Input: dimensioned drawing with shaded views. Units: mm. Origin: part minimum x, y, z. Coordinates: 2 decimals unless noted, no trailing zeros. Loops run counter-clockwise (first coordinate to the right, second up) from the corner with the lowest first, then second, coordinate; pieces in that order, holes last. Notation, with made-up numbers: M 27.25,58.5 L 81.25,58.5 A17 ccw 81.25,68.5 Z; hole C 47,17.25 d8. An arc over 180 degrees is marked long. Write item = value, one per line. Start each with the question number.
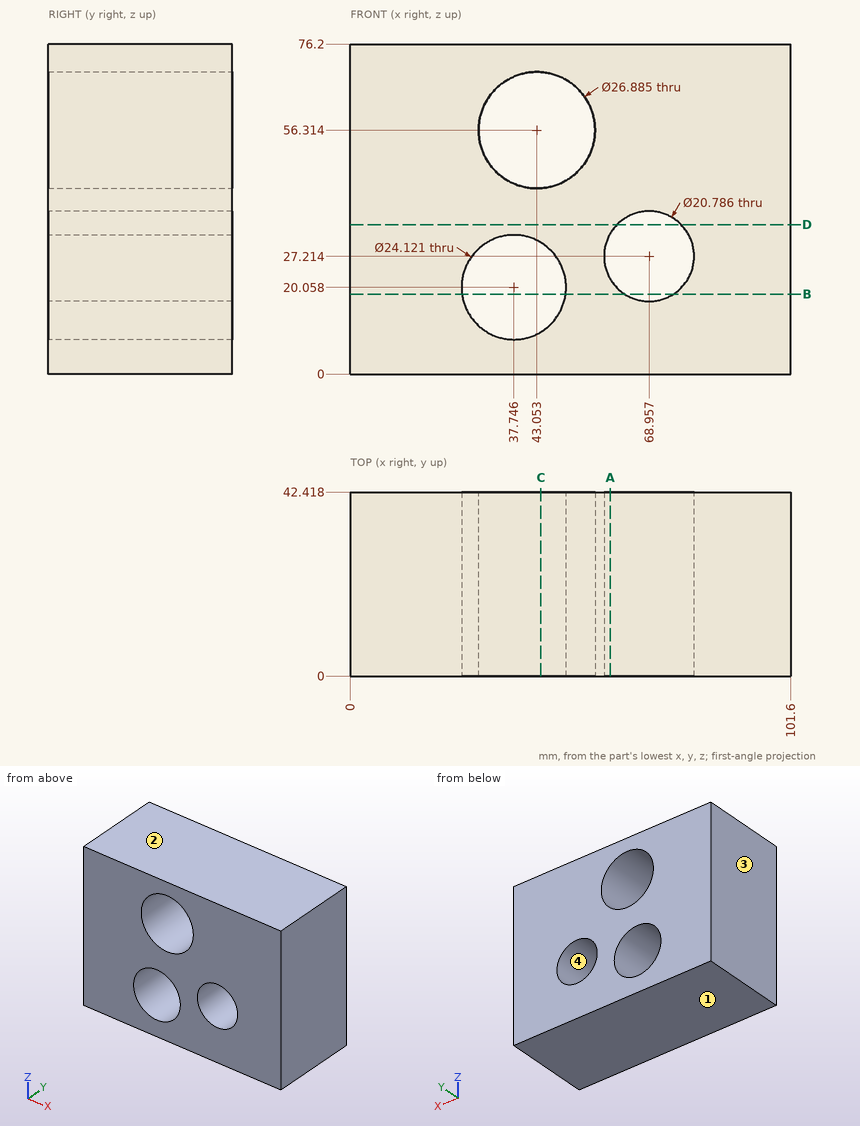
Item 1: Pull-direction query (Z, two-part tool) for the marked faces 1, 2, 3 and 4; classes: released by +Z, released by -Z, zero draft, split by the parting line, or undercut.
Item 2: Section query A-A (x = 60). Return the cut outline in (y, z) (1 decimal).
Item 3: Section query D-D (z = 34.5). Return the cut outline in (x, y), plus the area to 3 significant figures.
Item 4: First-contact query: pin 1 (3 mm diameter, centred on y = 34, z = 63, fed in from -X). Flat tip, straight axial feed; report the tip coordinate or a pass-through.
Item 5: Section query B-B (z = 18.5). Return the cut outline in (x, y) (1 decimal).
Item 6: Line query: line 1 (X direction, y = 11.5, z = 57); line 2 (X direction, y = 14.5, z = 21) (1 decimal); line 3 (Z direction, x = 46.5, y = 25) (1 decimal). Output: solid intervals per line, ascending. Write a range as from..to.
Item 7: Section query C-C (x = 44). Return the cut outline in (y, z) (1 decimal).
Verdict:
q1.face_1 = released by -Z
q1.face_2 = released by +Z
q1.face_3 = zero draft
q1.face_4 = undercut
q2.outline = M 0,0 L 42.4,0 L 42.4,21.9 L 0,21.9 Z; M 0,32.5 L 42.4,32.5 L 42.4,76.2 L 0,76.2 Z
q3.outline = M 0,0 L 61.55,0 L 61.55,42.42 L 0,42.42 Z; M 76.37,0 L 101.6,0 L 101.6,42.42 L 76.37,42.42 Z
q3.area = 3,680 mm2
q4.pin_1 = 0
q5.outline = M 0,0 L 25.8,0 L 25.8,42.4 L 0,42.4 Z; M 49.7,0 L 63.3,0 L 63.3,42.4 L 49.7,42.4 Z; M 74.6,0 L 101.6,0 L 101.6,42.4 L 74.6,42.4 Z
q6.line_1 = 0..29.63, 56.48..101.6
q6.line_2 = 0..25.7, 49.8..60.6, 77.3..101.6
q6.line_3 = 0..11.8, 28.4..43.3, 69.3..76.2
q7.outline = M 0,0 L 42.4,0 L 42.4,9.7 L 0,9.7 Z; M 0,30.4 L 42.4,30.4 L 42.4,42.9 L 0,42.9 Z; M 0,69.7 L 42.4,69.7 L 42.4,76.2 L 0,76.2 Z
